from build123d import *

# Parameters (mm, degrees)
PAD001_DEPTH = 9
SKETCH_R     = 4.5
PAD_DEPTH    = 19


with BuildPart() as pad001:
    # Sketch001 → Pad001 (new body)
    with BuildSketch(Plane.XY.offset(5)):
        Polygon((14.06139, 14.951333), (13.372483, -1.222209), (24.294571, -10.485819), (31.779444, -19.545599), (34.910954, 3.534533), align=None)
    extrude(amount=PAD001_DEPTH)


with BuildPart() as cut:
    # Sketch → Pad (new body)
    with BuildSketch(Plane.XY):
        with BuildLine():
            ThreePointArc((21.042951, 5.555957), (1.73939, 11.668843), (-17.564171, 5.555957))
            ThreePointArc((-17.564171, 5.555957), (-20.279768, -3.182793), (-12.525617, -8.042151))
            ThreePointArc((-12.525617, -8.042151), (-11.161352, -6.565238), (-12.474374, -5.042589))
            ThreePointArc((-13.247026, -0.576927), (-14.504081, -3.094097), (-12.474374, -5.042589))
            ThreePointArc((3.652051, 4.078635), (-5.036131, 2.617099), (-13.247026, -0.576927))
            ThreePointArc((9.233633, -0.919481), (7.491779, 2.750964), (3.652051, 4.078635))
            ThreePointArc((9.233633, -0.919481), (20.331777, -7.15317), (21.042951, 5.555957))
        make_face()
        with Locations((16.725806, -0.576927)):
            Circle(SKETCH_R, mode=Mode.SUBTRACT)
    extrude(amount=PAD_DEPTH)

    # Cut: cut Pad001
    add(pad001.part, mode=Mode.SUBTRACT)


solid = cut.part
Can you work these out from the model? Positions are in its coordinate system, mm. A direction names the side the tool comes from. Give positions to 0.01 mm unless a question says otherwise; leave off trailing zeros. Loops run counter-clockwise (first coordinate to the right, second up) from the corner with the lowest first, then second, coordinate; pieces in that order, holes last. Notation, with made-up numbers: (-36.75, -13) - (11.25, -13) arc R16 cw to (11.25, -9) - close; hole circle Ø11 at (88, 63). An arc over 180 degrees is marked (long way). Answer as a JSON object with one key per item and string values.
Q1. Imagine slicing it at A-A on z = 1.5. Write out the boundary of the cut face in (x, y).
Geometry says:
{"outline": "(-17.56, 5.56) arc R7.5 ccw to (-12.53, -8.04) arc R1.51 ccw to (-12.47, -5.04) arc R2.37 cw to (-13.25, -0.58) arc R43.19 cw to (3.65, 4.08) arc R5.25 cw to (9.23, -0.92) arc R7.5 ccw (long way) to (21.04, 5.56) arc R33.54 ccw to start; hole circle Ø9 at (16.73, -0.58)"}
Q2. Imagine slicing it at D-D on z = 9. Write out the boundary of the cut face in (x, y), plus the area to 3 significant figures.
Geometry says:
{"outline": "(-17.56, 5.56) arc R7.5 ccw to (-12.53, -8.04) arc R1.51 ccw to (-12.47, -5.04) arc R2.37 cw to (-13.25, -0.58) arc R43.19 cw to (3.65, 4.08) arc R5.25 cw to (9.23, -0.92) arc R7.5 ccw to (20.35, -7.14) - (17.77, -4.95) arc R4.5 cw to (13.54, 2.6) - (13.83, 9.42) arc R33.54 ccw to start", "area": "358 mm²"}
Q3. Imagine slicing it at C-C on y = -4.5. Write out the boundary of the cut face in (x, z), plus the area to 3 significant figures.
Geometry says:
{"outline": "(-19.64, 0) - (-13.7, 0) - (-13.7, 19) - (-19.64, 19) - close; (10.33, 0) - (14.52, 0) - (14.52, 19) - (10.33, 19) - close; (18.93, 0) - (23.12, 0) - (23.12, 5) - (18.93, 5) - close; (18.93, 14) - (23.12, 14) - (23.12, 19) - (18.93, 19) - close", "area": "234 mm²"}
Q4. Imagine slicing it at B-B on x = 19. Write out the boundary of the cut face in (y, z).
Geometry says:
{"outline": "(-7.72, 0) - (-4.46, 0) - (-4.46, 5) - (-6, 5) - (-6, 14) - (-4.46, 14) - (-4.46, 19) - (-7.72, 19) - close; (3.31, 0) - (6.89, 0) - (6.89, 5) - (3.31, 5) - close; (3.31, 14) - (6.89, 14) - (6.89, 19) - (3.31, 19) - close"}
Q5. If we mould it in two halves opening along Y, with no side actions, what happens to faces 1 (the cylindrical face through (-20.326, -3.053, 9.367)), 2 (the flat face through (13.682, 6.053, 9.437)), 3 (the flat face through (1, 4, 19))? For each: pulls with the +Y half, pulls with the -Y half, needs draft (parallel to the pull), parting line crosses it, or undercut.
Geometry says:
{"face 1": "parting line crosses it", "face 2": "undercut", "face 3": "needs draft"}
Q6. If I drill on L1, parallel to Z at x = 20.5, y = -3.75; L2, parallel to X at y = 0.5, z = 4.5; L3, parallel to X at y = -0.25, z = 14.5, over which ranges is the centre line in solid material (lowest first)?
Geometry says:
{"L1": "0 to 5, 14 to 19", "L2": "-20.67 to -10.98, 8.97 to 12.36, 21.1 to 24.15", "L3": "-20.74 to -12.59, 9.16 to 12.24, 21.21 to 24.22"}
Q7. Which directions (+Z, -Z, +X, -X, +Y, -Y) give clear straight access to the entire face, cutting with the end or side of a thin tool? Please do faces 4 (the cylindrical face through (-11.162, -6.596, 9.367)), 5 (the flat face through (19.04, -6.03, 9.44)), 6 (the cylindrical face through (7.535, 2.712, 9.367)).
Geometry says:
{"face 4": "+Z, -Z", "face 5": "+X, +Y", "face 6": "+Z, -Z, -Y"}
Q8. Will these pins go through, and if not, where does the flat tip stop? P1, Ø1.5, axis at x = -15.5, z = 2.5, coming from the -Y side; P2, Ø1.5, axis at y = 1, z = 15.5, coming from the +X side; P3, Ø1.5, axis at x = -4, z = 11, coming from the -Y side.
Geometry says:
{"P1": "y = -7.92", "P2": "x = 24.18", "P3": "y = 2.69"}
